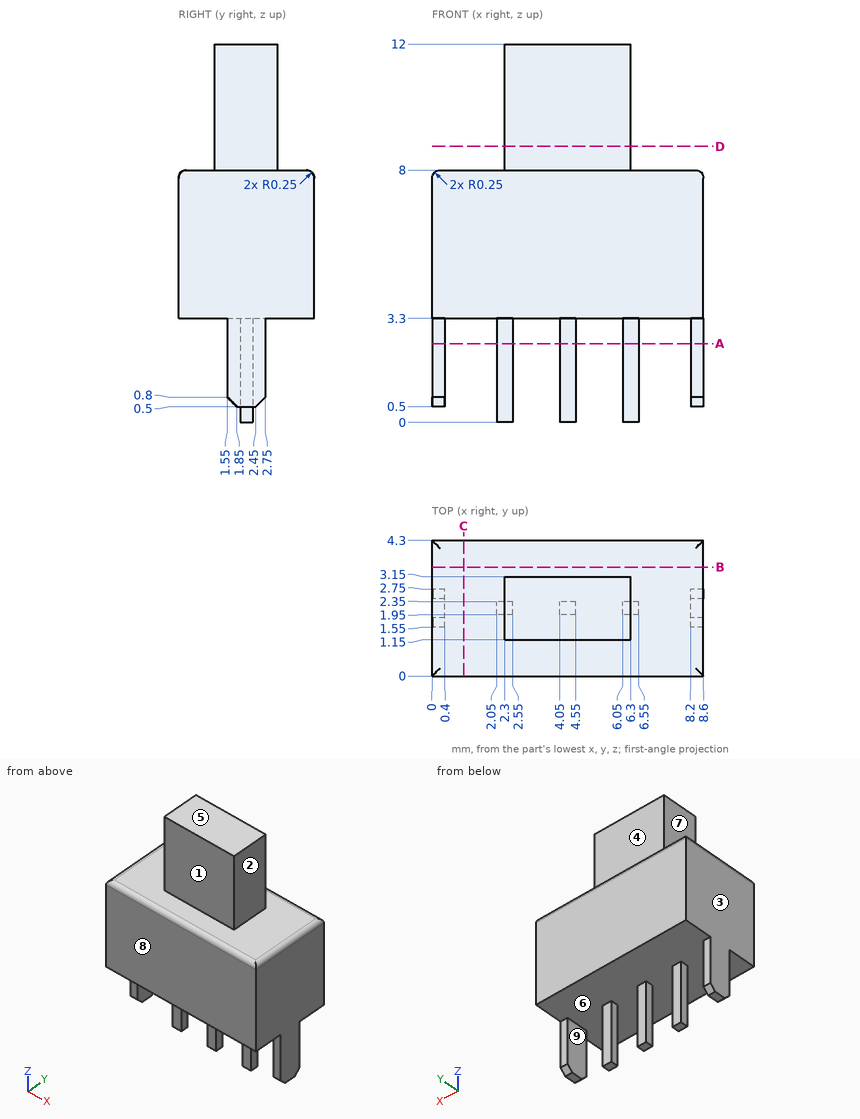
Print and shaded views of the part. All mm, measured from the part's lowest x, y and z. A direction names the side the tool comes from. Round coordinates to 2 decimals unless told otherwise and drop trailing zeros. Write each loop counter-clockwise with the first axis right and the second up, starting at its lowest first coordinate (ties: lowest second). Pieces come first, ordered by that corner, then holes. Notation, with made-up numbers: (-1, -2.75) -> (49, -2.75) arc R22 ccw to (49, 32.25) -> close; hole circle Ø1 at (63, 56). An arc over 180 degrees is marked (long way). Answer in a Markdown table with one row per item. Add a question column.
Item 1: Drop flat-ended pins along their axis: pin 1 Ø3 at (x, z) = (6, 8) entering from +Y; pin 2 Ø2 at (x, y) = (3.5, 4) entering from -Z; pin 3 Ø0.6 at (x, z) = (6.5, 2) entering from -Y; pin 4 Ø1 at (y, z) = (2, 10) entering from -X. Give the stop position or say it passes through.
Item 2: Saw through at A-A, the plane z = 2.5. Write the cut outline in (x, y).
Item 3: Saw through at B-B, the plane y = 3.45. Write the cut outline in (x, z).
Item 4: Mould opens along X. For the marked faces 6, 7, 8 and 9 say: pulls with the +X half, pulls with the -X half, needs draft (parallel to the pull), parting line crosses it, or undercut.
Item 5: Saw through at D-D, the plane z = 8.75. Write the cut outline in (x, y), then the cut area to 3 significant figures.
Item 6: Saw through at C-C, the plane x = 1. Write the cut outline in (y, z), then the cut area to 3 significant figures.
Item 7: Which spindle directions (+Z, -Z, +X, -X, +Y, -Y) get a long thin tool onto all of the face, cutting with end or side? Do the marked faces 1, 2, 3, 4 and 5. Say none if no direction does.
Item 8: Drill centre lines: line 1 (Z direction, x = 3.25, y = 1); line 2 (Y direction, x = 6, z = 9.75); line 3 (Z direction, x = 3, y = 1.7). Where is each one in solid material? Low to high. Write a range as from..to.
Findings below:
| question | item | result |
|---|---|---|
| 1 | pin 1 | stops at y = 4.3 |
| 1 | pin 2 | stops at z = 3.3 |
| 1 | pin 3 | stops at y = 1.95 |
| 1 | pin 4 | stops at x = 2.3 |
| 2 | outline | (0, 1.55) -> (0.4, 1.55) -> (0.4, 2.75) -> (0, 2.75) -> close; (2.05, 1.95) -> (2.55, 1.95) -> (2.55, 2.35) -> (2.05, 2.35) -> close; (4.05, 1.95) -> (4.55, 1.95) -> (4.55, 2.35) -> (4.05, 2.35) -> close; (6.05, 1.95) -> (6.55, 1.95) -> (6.55, 2.35) -> (6.05, 2.35) -> close; (8.2, 1.55) -> (8.6, 1.55) -> (8.6, 2.75) -> (8.2, 2.75) -> close |
| 3 | outline | (0, 3.3) -> (8.6, 3.3) -> (8.6, 7.75) arc R0.25 ccw to (8.35, 8) -> (0.25, 8) arc R0.25 ccw to (0, 7.75) -> close |
| 4 | face 6 | undercut |
| 4 | face 7 | pulls with the -X half |
| 4 | face 8 | needs draft |
| 4 | face 9 | undercut |
| 5 | outline | (2.3, 1.15) -> (6.3, 1.15) -> (6.3, 3.15) -> (2.3, 3.15) -> close |
| 5 | area | 8.00 mm^2 |
| 6 | outline | (0, 3.3) -> (4.3, 3.3) -> (4.3, 7.75) arc R0.25 ccw to (4.05, 8) -> (0.25, 8) arc R0.25 ccw to (0, 7.75) -> close |
| 6 | area | 20.2 mm^2 |
| 7 | face 1 | +Z, +X, -X, -Y |
| 7 | face 2 | +Z, +X, +Y, -Y |
| 7 | face 3 | +Z, -Z, -X, +Y, -Y |
| 7 | face 4 | +Z, +X, -X, +Y |
| 7 | face 5 | +Z, +X, -X, +Y, -Y |
| 8 | line 1 | z = 3.3..8 |
| 8 | line 2 | y = 1.15..3.15 |
| 8 | line 3 | z = 3.3..12 |
